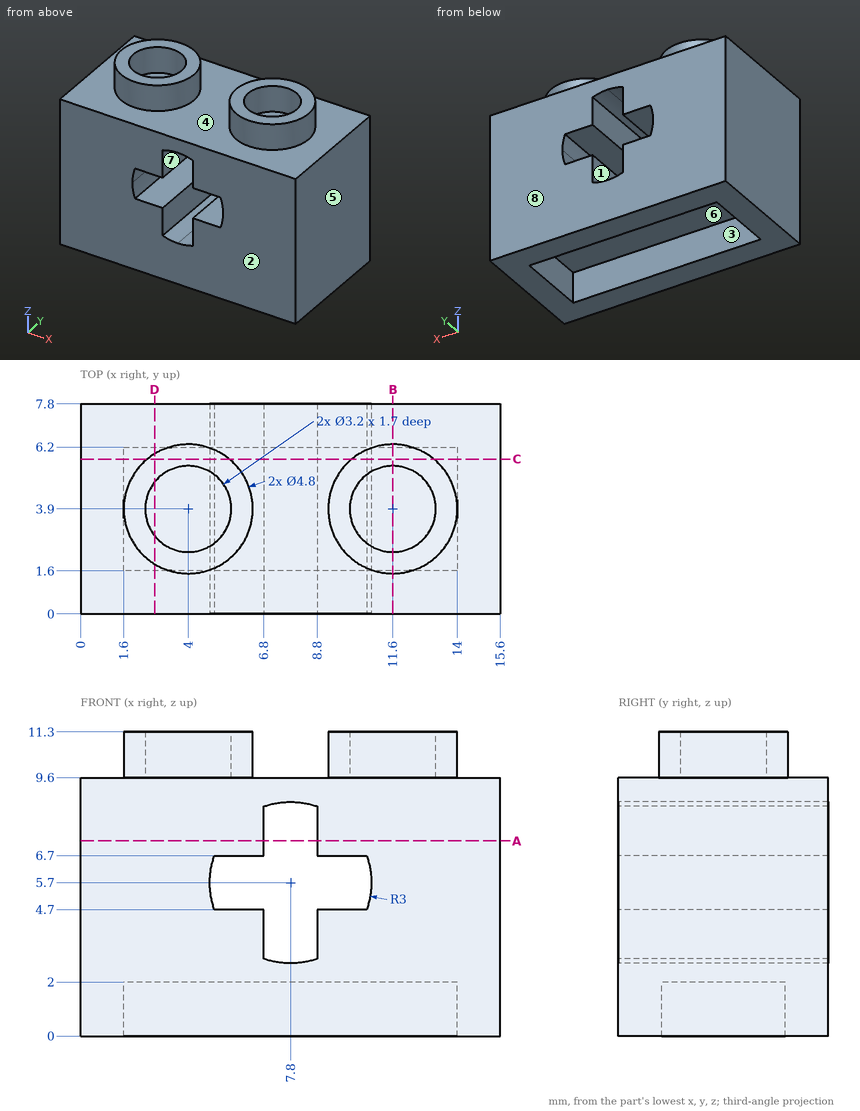
The figure shows three views and two pictorial views of one solid part (mm, origin at its lowest corner). Answer the questions. A direction names the side the tool comes from. Round coordinates to 2 decimals unless told otherwise and drop trailing zeros. Order: outer loops, then holes, each group sorted by start corner. A loop starts at its lowest first (then second) coordinate and runs counter-clockwise, first axis right, second up.
Q1. Find the intervals of material crossed by line 1 along X through (y, z) = (1, 8.5); line 2 along Z through (x, y) = (7.75, 0.75); line 3 along Y through (x, z) = (4, 10.55), in increasing order.
Solution:
line 1: x = 0 to 6.8, 8.8 to 15.6
line 2: z = 0 to 2.7, 8.7 to 9.6
line 3: y = 1.5 to 2.3, 5.5 to 6.3
Q2. The mould has two halves that part along Y. Classify the marked faces 6, 7 and 8: pulls with the +Y half, pulls with the -Y half, needs draft (parallel to the pull), parting line crosses it, or undercut.
Solution:
face 6: undercut
face 7: needs draft
face 8: pulls with the +Y half
Q3. Given pin 1 Ø0.9 at (x, y) = (6, 2) entering from +Z; pin 2 Ø4 at (x, y) = (11.6, 3.9) entering from -Z; pin 3 Ø1 at (x, y) = (4.5, 3.5) entering from +Z, each flat-ended and moving along its own axis, determine where each tip first touches the part or whether it passes through.
Solution:
pin 1: stops at z = 11.3
pin 2: stops at z = 2
pin 3: stops at z = 9.6
Q4. A cutting plane is placed at B-B, the plane x = 11.6. Determine the outline of the cut face in (y, z), then the cut area to 3 significant figures.
Solution:
outline: (0, 0) - (1.6, 0) - (1.6, 2) - (6.2, 2) - (6.2, 0) - (7.8, 0) - (7.8, 9.6) - (6.3, 9.6) - (6.3, 11.3) - (5.5, 11.3) - (5.5, 9.6) - (2.3, 9.6) - (2.3, 11.3) - (1.5, 11.3) - (1.5, 9.6) - (0, 9.6) - close
area: 68.4 mm2
Q5. A cutting plane is placed at C-C, the plane y = 5.75. Determine the outline of the cut face in (x, z).
Solution:
outline: (0, 0) - (1.6, 0) - (1.6, 2) - (14, 2) - (14, 0) - (15.6, 0) - (15.6, 9.6) - (13.13, 9.6) - (13.13, 11.3) - (10.07, 11.3) - (10.07, 9.6) - (5.53, 9.6) - (5.53, 11.3) - (2.47, 11.3) - (2.47, 9.6) - (0, 9.6) - close; hole (4.97, 4.7) - (6.8, 4.7) - (6.8, 2.87) arc R3 ccw to (8.8, 2.87) - (8.8, 4.7) - (10.63, 4.7) arc R3 ccw to (10.63, 6.7) - (8.8, 6.7) - (8.8, 8.53) arc R3 ccw to (6.8, 8.53) - (6.8, 6.7) - (4.97, 6.7) arc R3 ccw to start
Q6. A cutting plane is placed at A-A, the plane z = 7.25. Determine the outline of the cut face in (x, y).
Solution:
outline: (0, 0) - (6.8, 0) - (6.8, 7.8) - (0, 7.8) - close; (8.8, 0) - (15.6, 0) - (15.6, 7.8) - (8.8, 7.8) - close
Q7. A cutting plane is placed at D-D, the plane x = 2.75. Determine the outline of the cut face in (y, z).
Solution:
outline: (0, 0) - (1.6, 0) - (1.6, 2) - (6.2, 2) - (6.2, 0) - (7.8, 0) - (7.8, 9.6) - (5.95, 9.6) - (5.95, 11.3) - (4.9, 11.3) - (4.9, 9.6) - (2.9, 9.6) - (2.9, 11.3) - (1.85, 11.3) - (1.85, 9.6) - (0, 9.6) - close
Q8. A tool of negligible diameter and unlimited length cuts with its end or side. For the marked faces 1, 2, 3, 4 and 5, from which of +Z, -Z, +X, -X, +Y, -Y can it reach the whole face along a straight path? Write none if from no direction.
Solution:
face 1: +Y, -Y
face 2: +Z, -Z, +X, -X, -Y
face 3: -Z
face 4: +Z
face 5: +Z, -Z, +X, +Y, -Y
